from build123d import *

# Parameters (mm, degrees)
SKETCH1_R           = 1.5
BOSS_EXTRUDE1_DEPTH = 9.75
SKETCH3_R           = 1.675
CUT_EXTRUDE1_DEPTH  = 10
CUT_EXTRUDE2_REACH  = 64.002
SKETCH1_4_R         = 8
FILLET1_R           = 3.25
SKETCH1_5_R         = 15.1375
SKETCH1_5_R_2       = 8
CUT_EXTRUDE3_DEPTH  = 8.75


with BuildPart() as part:
    # Sketch1 → Boss-Extrude1 (new body)
    with BuildSketch(Plane(origin=(0, 0, 0), x_dir=(0, 0, -1), z_dir=(1, 0, 0))):
        with BuildLine():
            Line((20.1375, 0), (20.1375, 43.3))
            Line((20.1375, 43.3), (30.1375, 43.3))
            Line((30.1375, 43.3), (30.1375, 53.3))
            Line((30.1375, 53.3), (-30.1375, 53.3))
            Line((-30.1375, 53.3), (-30.1375, 43.3))
            Line((-30.1375, 43.3), (-20.1375, 43.3))
            Line((-20.1375, 43.3), (-20.1375, 0))
            ThreePointArc((-20.1375, 0), (0, -20.1375), (20.1375, 0))
        make_face()
        Polygon((-17.1375, 38.810813136), (-2.327943822, 26.332666354), (-17.1375, 13.854519572), align=None, mode=Mode.SUBTRACT)
        with Locations((-12.43443714, 48.8)):
            Circle(SKETCH1_R, mode=Mode.SUBTRACT)
        with Locations((0, 22.254350724)):
            Circle(SKETCH1_R, mode=Mode.SUBTRACT)
        Polygon((2.327943822, 26.332666354), (17.1375, 38.810813136), (17.1375, 13.854519572), align=None, mode=Mode.SUBTRACT)
        Polygon((0, 28.294131259), (-16.171581688, 41.919885304), (0, 49.950465907), (16.171581688, 41.919885304), align=None, mode=Mode.SUBTRACT)
        with Locations((12.43443714, 48.8)):
            Circle(SKETCH1_R, mode=Mode.SUBTRACT)
    extrude(amount=BOSS_EXTRUDE1_DEPTH)

    # Sketch3 → Cut-Extrude1 (cut)
    with BuildSketch(Plane(origin=(0, 53.3, 0), x_dir=(1, 0, 0), z_dir=(0, 1, 0))):
        with Locations(Location((4.875, 25.1375, 0), (0, 0, 270))):
            Circle(SKETCH3_R)
        with Locations(Location((4.875, -25.1375, 0), (0, 0, 90))):
            Circle(SKETCH3_R)
    extrude(amount=-CUT_EXTRUDE1_DEPTH, mode=Mode.SUBTRACT)

    # Sketch1<4> → Cut-Extrude2 (cut, up to next)
    with BuildSketch(Plane(origin=(0, 0, 0), x_dir=(0, 0, -1), z_dir=(1, 0, 0)), mode=Mode.PRIVATE) as cut_extrude2_sk1:
        Circle(SKETCH1_4_R)
    cut_extrude2_tool1 = extrude(cut_extrude2_sk1.sketch, amount=CUT_EXTRUDE2_REACH, mode=Mode.PRIVATE) & part.part
    add(cut_extrude2_tool1.solids().sort_by_distance((0, 0, 0))[0], mode=Mode.SUBTRACT)

    # Fillet1
    fillet1_edges = [part.edges().sort_by_distance(p)[0] for p in [
        (4.875, 41.919885304, -16.171581688),
        (4.875, 49.950465907, 0),
        (4.875, 41.919885304, 16.171581688),
        (4.875, 28.294131259, 0),
        (4.875, 38.810813136, 17.1375),
        (4.875, 13.854519572, 17.1375),
        (4.875, 26.332666354, 2.327943822),
        (4.875, 53.3, -30.1375),
        (4.875, 43.3, -30.1375),
        (4.875, 43.3, -20.1375),
        (4.875, 43.3, 20.1375),
        (4.875, 43.3, 30.1375),
        (4.875, 53.3, 30.1375),
        (4.875, 13.854519572, -17.1375),
        (4.875, 38.810813136, -17.1375),
        (4.875, 26.332666354, -2.327943822),
    ]]
    fillet(fillet1_edges, radius=FILLET1_R)

    # Sketch1<5> → Cut-Extrude3 (cut)
    with BuildSketch(Plane(origin=(0, 0, 0), x_dir=(0, 0, -1), z_dir=(1, 0, 0))):
        with Locations(Location((0, 0, 0), (0, 0, 180))):
            Circle(SKETCH1_5_R)
        Circle(SKETCH1_5_R_2, mode=Mode.SUBTRACT)
    extrude(amount=CUT_EXTRUDE3_DEPTH, mode=Mode.SUBTRACT)


solid = part.part
Can you work these out from the model? Positions are in its coordinate system, mm. A direction names the side the tool comes from. Round coordinates to 2 decimals unless told otherwise and drop trailing zeros. Loops run counter-clockwise (first coordinate to the right, second up) from the corner with the lowest first, then second, coordinate; pieces in that order, holes last. Notation, with made-up numbers: (47.5, 54.25) - (76.5, 54.25) arc R24 ccw to (76.5, 86.25) - close; hole circle Ø2 at (21.5, 54). An arc over 180 degrees is marked (long way). Answer in a Markdown table with one row per item. Add a question column.
Q1. I want a section at C-C on y = -13. List the corners of the cut face in (x, z) for me, and give its area (3 significant figures).
Q2. We'd pull the mould along Z, two halves only. Please class faces 1 (the cylindrical face through (4.807, -20.133, 0.443)), 2 (the flat face through (4.81, 21.14, 8.49)), 3 (the flat face through (4.81, 31.6, 8.58)), 4 (the flat face through (5, 48, 30.138)): pulls with the +Z half, pulls with the -Z half, needs draft (parallel to the pull), parting line crosses it, or undercut.
Q3. I want a section at D-D on z = 25. List the corners of the cut face in (x, y) for me.
Q4. Which directions (+Z, -Z, +X, -X, +Y, -Y) give clear straight access to the entire face, cutting with the end or side of a thin tool? Please do faces 5 (the cylindrical face through (4.94, 49.57, -0.02)), 6 (the flat face through (9.75, 17, 0)), 7 (the cylindrical face through (4.95, 48.37, -26.81)), 8 (the cylindrical face through (4.31, -15.01, -1.97)), 9 (the flat face through (5, 20, 20.138)).
Q5. I need wall thicknesses on L1, parallel to Y at x = 2.5, z = 0; L2, parallel to Z at x = 6.5, y = 26.5; L3, parallel to Y at x = 2.5, z = 1. Which ranges of each line are inside material? Lowest first, please.
Q6. I want a section at A-A on z = 0. List the corners of the cut face in (x, y) for me.
Q7. For pin 1 Ø13 at (y, z) = (0, 0) entering from -X; pin 2 Ø5 at (x, y) = (6.5, 23.5) entering from +Z; pin 3 Ø3 at (x, y) = (6.5, 32.5) entering from -Z; pin 4 Ø3 at (x, z) = (6, -6) entering from -Y, each with a flat end and sliding along its axis, tell me the tip position at first contact or that it passes through.
Q8. I want a section at B-B on y = -3.5. List the corners of the cut face in (x, z) for me, and give its area (3 significant figures).
A:
| question | item | result |
|---|---|---|
| 1 | outline | (0, -15.38) - (9.75, -15.38) - (9.75, 15.38) - (0, 15.38) - (0, 7.76) - (8.75, 7.76) - (8.75, -7.76) - (0, -7.76) - close |
| 1 | area | 164 mm^2 |
| 2 | face 1 | parting line crosses it |
| 2 | face 2 | undercut |
| 2 | face 3 | undercut |
| 2 | face 4 | pulls with the +Z half |
| 3 | outline | (0, 43.3) - (3.21, 43.3) - (3.21, 53.3) - (0, 53.3) - close; (6.54, 43.3) - (9.75, 43.3) - (9.75, 53.3) - (6.54, 53.3) - close |
| 4 | face 5 | +X, -X |
| 4 | face 6 | +Z, -Z, +X, +Y, -Y |
| 4 | face 7 | +Y, -Y |
| 4 | face 8 | -X |
| 4 | face 9 | +Z, +X, -X, -Y |
| 5 | L1 | -20.14 to -15.14, 15.14 to 20.75, 23.75 to 29.29, 49.57 to 53.3 |
| 5 | L2 | -20.14 to -17.14, -4.13 to 4.13, 17.14 to 20.14 |
| 5 | L3 | -20.11 to -15.1, 15.1 to 21.14, 23.37 to 29.45, 49.41 to 53.3 |
| 6 | outline | (0, -20.14) - (9.75, -20.14) - (9.75, -8) - (8.75, -8) - (8.75, -15.14) - (0, -15.14) - close; (0, 15.14) - (8.75, 15.14) - (8.75, 8) - (9.75, 8) - (9.75, 20.75) - (0, 20.75) - close; (0, 23.75) - (9.75, 23.75) - (9.75, 29.29) - (0, 29.29) - close; (0, 49.57) - (9.75, 49.57) - (9.75, 53.3) - (0, 53.3) - close |
| 7 | pin 1 | through |
| 7 | pin 2 | z = 20.14 |
| 7 | pin 3 | z = -20.14 |
| 7 | pin 4 | y = -19.63 |
| 8 | outline | (0, -19.83) - (9.75, -19.83) - (9.75, -7.19) - (8.75, -7.19) - (8.75, -14.73) - (0, -14.73) - close; (0, 14.73) - (8.75, 14.73) - (8.75, 7.19) - (9.75, 7.19) - (9.75, 19.83) - (0, 19.83) - close |
| 8 | area | 115 mm^2 |
